```python
from build123d import *

# Parameters (mm, degrees)
ESQUISSE1_W             = 330
ESQUISSE1_H             = 180
BOSS_EXTRU_1_DEPTH      = 6
ESQUISSE2_W             = 40
ESQUISSE2_H             = 6
ESQUISSE2_H_2           = 9.903585907
ENL_V_MAT_ENCOCHE_DEPTH = 6
ESQUISSE3_R             = 8
ESQUISSE3_W             = 15
ESQUISSE3_H             = 29
ESQUISSE3_W_2           = 8
ESQUISSE3_H_2           = 20
ENL_V_MAT_EXTRU_1_DEPTH = 10


with BuildPart() as part:
    # Esquisse1 → Boss.-Extru.1 (new body)
    with BuildSketch(Plane.XY):
        with Locations((-165, 90)):
            Rectangle(ESQUISSE1_W, ESQUISSE1_H)
    extrude(amount=BOSS_EXTRU_1_DEPTH)

    # Esquisse2 → Enlèv. mat encoche (cut)
    with BuildSketch(Plane.XY.offset(6)):
        with Locations((-245, 177)):
            Rectangle(ESQUISSE2_W, ESQUISSE2_H)
        with Locations((-165, 177)):
            Rectangle(ESQUISSE2_W, ESQUISSE2_H)
        with Locations((-85, 177)):
            Rectangle(ESQUISSE2_W, ESQUISSE2_H)
        with Locations((-245, 4.951792954)):
            Rectangle(ESQUISSE2_W, ESQUISSE2_H_2)
        with Locations((-165, 4.951792954)):
            Rectangle(ESQUISSE2_W, ESQUISSE2_H_2)
        with Locations((-85, 4.951792954)):
            Rectangle(ESQUISSE2_W, ESQUISSE2_H_2)
    extrude(amount=-ENL_V_MAT_ENCOCHE_DEPTH, mode=Mode.SUBTRACT)

    # Esquisse3 → Enlèv. mat.-Extru.1 (cut)
    with BuildSketch(Plane.XY.offset(6)):
        with Locations((-40, 25)):
            Circle(ESQUISSE3_R)
        with Locations((-95.5, 30.5)):
            Rectangle(ESQUISSE3_W, ESQUISSE3_H)
        with Locations((-64, 26)):
            Rectangle(ESQUISSE3_W_2, ESQUISSE3_H_2)
    extrude(amount=-ENL_V_MAT_EXTRU_1_DEPTH, mode=Mode.SUBTRACT)


solid = part.part
```
For this review, take the finished solid that the model builds, in its own axes (mm). A direction names the side the tool comes from. Give positions to 0.01 mm unless a question says otherwise; leave off trailing zeros. Loops run counter-clockwise (first coordinate to the right, second up) from the corner with the lowest first, then second, coordinate; pieces in that order, holes last. Notation, with made-up numbers: M 81.25,2 L 129.25,2 A33 cw 129.25,41 Z; hole C 56,-33.75 d6. An arc over 180 degrees is marked long. One line per item, written item: value. Start each with the question number.
Q1. Clearance check with a flat-ended pin moving along its axis: pin 1 Ø2 at (x, z) = (-101, 1.5) entering from +Y. State where the tip first meets the part, or that it passes through.
Q2. For L1, parallel to Y at x = -40, z = 1.75; L2, parallel to X at y = 27, z = 1.1; L3, parallel to X at y = 38, z = 5.05, list the stretches that pass through material, from the lowest coordinate up.
Q3. Machinability: for faces 3 (the face through (-68, 26, 3)), 4 (the face through (-105, 5, 3)), 5 (the face through (-225, 177, 3)), 6 (the face through (-125, 0, 3)), which of the approach directions +Z, -Z, +X, -X, +Y, -Y give a long, thin tool a straight path to every point of the face, cutting with its end or side? Answer none if there is none.
Q4. Add section B-B (y = 25). Give the boundary of the cut face in (x, z).
Q5. Draft analysis for pull direction X (two halves, no side actions). For faces 1 (the face through (-85, 174, 3)), 2 (the face through (-33, 180, 3)), state which applies: released by +X, released by -X, zero draft, split by the parting line, or undercut.
Q6. Add section C-C (z = 4.7). Count the separate pieces of the cut face and the enclosed holes in it, and give its area (3 significant figures).
Q7. Add section A-A (x = -40). Give the boundary of the cut face in (y, z), and give its area (3 significant figures).
Reply:
1. pin 1: y = 174
2. L1: 0 to 17, 33 to 180
2. L2: -330 to -103, -88 to -68, -60 to -47.75, -32.25 to 0
2. L3: -330 to -103, -88 to 0
3. face 3: +Z, -Z
3. face 4: +Z, -Z, -Y
3. face 5: +Z, -Z, +Y
3. face 6: +Z, -Z, +X, -X, -Y
4. outline: M -330,0 L -103,0 L -103,6 L -330,6 Z; M -88,0 L -68,0 L -68,6 L -88,6 Z; M -60,0 L -48,0 L -48,6 L -60,6 Z; M -32,0 L 0,0 L 0,6 L -32,6 Z
5. face 1: undercut
5. face 2: zero draft
6. separate pieces: 1
6. enclosed holes: 3
6. area: 56,700 mm²
7. outline: M 0,0 L 17,0 L 17,6 L 0,6 Z; M 33,0 L 180,0 L 180,6 L 33,6 Z
7. area: 984 mm²
